Work out the finished part from the listing and answer in its coordinate system (mm). Face numbers are marked on the shaded views. A direction names the side the tool comes from. Coordinates: 2 decimals unless noted, no trailing zeros. Order: outer loops, then holes, each group sorted by start corner. A loop starts at its lowest first (then second) coordinate and runs counter-clockwise, first axis right, second up. Notation, with made-up numbers: (-31, 87) -> (28, 87) arc R25 cw to (28, 105) -> close; hole circle Ø3 at (35.25, -39.5). An arc over 180 degrees is marked (long way). Use one line per item in the form item = value.
Autodesk Inventor part; units mm, degrees
ref_plane "YZ Plane" through (0, 0, 0) normal (1, 0, 0) x (0, 1, 0)
ref_plane "XZ Plane" through (0, 0, 0) normal (0, 1, 0) x (-1, 0, 0)
ref_plane "XY Plane" through (0, 0, 0) normal (0, 0, 1) x (1, 0, 0)
sketch "Sketch1" plane through (0, 0, 0) normal (0, 1, 0) x (-1, 0, 0)
  circle A0 centre (0, 0) radius 47.5
  dimension "d0" = 95
extrude "Extrusion1" add sketch "Sketch1" along normal blind 6
sketch "Sketch2" plane through (0, 6, 0) normal (0, 1, 0) x (1, 0, 0)
  circle A0 centre (0, 0) radius 10
  circle A1 centre (0, 5) radius 1
  circle A2 centre (0, -5) radius 1
  dimension "d3" = 20
  dimension "d4" = 2
  dimension "d5" = 2
extrude "Extrusion2" cut sketch "Sketch2" against normal blind 23.4625 contours A1 | A2
sketch "Sketch4" plane through (0, 6, 0) normal (0, 1, 0) x (1, 0, 0)
  line L0 (0, 0) -> (-10, 0)
  line L1 (-10, 0) -> (-10, 25)
  line L2 (-10, 25) -> (0, 25)
  line L3 (0, 25) -> (0, 0)
  line L4 (0, 0) -> (-5, 0)
  line L5 (-5, 0) -> (-5, 25)
  line L6 (-5, 25) -> (0, 25)
  line L7 (0, 25) -> (0, 0)
  line L8 (-5, 25) -> (-20, 25)
  line L9 (-20, 25) -> (-20, -25)
  line L10 (-20, -25) -> (-5, -25)
  line L11 (-5, -25) -> (-5, 25)
  line L12 (-5, 25) -> (-25, 25)
  line L13 (-25, 25) -> (-25, -25)
  line L14 (-25, -25) -> (-5, -25)
  line L15 (-5, -25) -> (-5, 25)
  dimension "d9" = 10
  dimension "d10" = 25
  dimension "d11" = 15
  dimension "d12" = 50
  dimension "d13" = 20
extrude "Extrusion3" add sketch "Sketch4" along normal blind 70 contours L11 L10 L9 L8 L1 L0 | L0 L1 L2 L5 | L14 L13 L12 L9
sketch "Sketch5" plane through (-25, 6, -25) normal (-1, 0, 0) x (0, 0, 1)
  line L0 (0, 0) -> (0, 70)
  line L1 (50, 0) -> (50, 70)
  line L2 (0, 70) -> (50, 70)
  line L3 (50, 70) -> (50, 0)
  line L4 (50, 0) -> (0, 0)
  line L5 (0, 0) -> (0, 70)
  line L6 (50, 70) -> (0, 70)
  line L7 (72.5, 0) -> (-22.5, 0)
  line L8 (0, 70) -> (25, 70)
  line L9 (25, 70) -> (25, 0)
  line L10 (25, 0) -> (0, 0)
  line L11 (0, 0) -> (0, 70)
  line L12 (25, 35) -> (15, 35)
  line L13 (15, 35) -> (15, 15)
  line L14 (15, 15) -> (25, 15)
  line L15 (25, 15) -> (25, 35)
  line L16 (15, 35) -> (25, 35)
  line L17 (25, 35) -> (25, 55)
  line L18 (25, 55) -> (15, 55)
  line L19 (15, 55) -> (15, 35)
  line L20 (15, 15) -> (35, 15)
  line L21 (35, 15) -> (35, 55)
  line L22 (35, 55) -> (15, 55)
  line L23 (15, 55) -> (15, 15)
  line L24 (15, 15) -> (35, 15)
  line L25 (35, 15) -> (35, 55.5)
  line L26 (35, 55.5) -> (15, 55.5)
  line L27 (15, 55.5) -> (15, 15)
  point P0 (25, -6)
  dimension "d16" = 10
  dimension "d17" = 20
  dimension "d18" = 20
  dimension "d19" = 20
  dimension "d20" = 40.5
extrude "Extrusion4" cut sketch "Sketch5" against normal blind 16 contours L14 L13 L12 L9 | L9 L22 L21 L20 | L26 L25 L22 L9 | L9 L18 L27 L26 | L12 L19 L18 L9
sketch "Sketch6" plane through (-25, 6, -25) normal (-1, 0, 0) x (0, 0, 1)
  line L0 (35, 15) -> (15, 15)
  line L1 (15, 15) -> (35, 15)
  line L2 (35, 15) -> (35, 9)
  line L3 (35, 9) -> (15, 9)
  line L4 (15, 9) -> (15, 15)
  line L5 (15, 55.5) -> (35, 55.5)
  line L6 (15, 55.5) -> (35, 55.5)
  line L7 (35, 55.5) -> (35, 61.5)
  line L8 (35, 61.5) -> (15, 61.5)
  line L9 (15, 61.5) -> (15, 55.5)
  point P0 (25, -6)
  dimension "d23" = 6
  dimension "d24" = 6
extrude "Extrusion5" cut sketch "Sketch6" against normal blind 6
sketch "Sketch7" plane through (-19, 6, -25) normal (-1, 0, 0) x (0, 0, 1)
  line L0 (35, 9) -> (15, 9)
  line L1 (35, 61.5) -> (35, 9)
  line L2 (15, 9) -> (35, 9)
  line L3 (35, 9) -> (35, 11.6)
  line L4 (35, 11.6) -> (15, 11.6)
  line L5 (15, 11.6) -> (15, 9)
  line L6 (15, 55.5) -> (15, 61.5)
  line L7 (35, 61.5) -> (35, 55.5)
  line L8 (15, 61.5) -> (35, 61.5)
  line L9 (35, 61.5) -> (35, 58.5)
  line L10 (35, 58.5) -> (15, 58.5)
  line L11 (15, 58.5) -> (15, 61.5)
  line L12 (15, 9) -> (15, 61.5)
  line L13 (15, 9) -> (35, 9)
  line L14 (35, 9) -> (35, 12)
  line L15 (35, 12) -> (15, 12)
  line L16 (15, 12) -> (15, 9)
  line L17 (35, 15) -> (15, 15)
  line L18 (25, 15) -> (20, 15)
  line L19 (20, 15) -> (20, 12)
  line L20 (20, 12) -> (25, 12)
  line L21 (25, 12) -> (25, 15)
  line L22 (25, 15) -> (30, 15)
  line L23 (30, 15) -> (30, 12)
  line L24 (30, 12) -> (25, 12)
  line L25 (25, 12) -> (25, 15)
  line L26 (15, 61.5) -> (35, 61.5)
  line L27 (25, 58.5) -> (20, 58.5)
  line L28 (20, 58.5) -> (20, 61.5)
  line L29 (20, 61.5) -> (25, 61.5)
  line L30 (25, 61.5) -> (25, 58.5)
  line L31 (25, 58.5) -> (30, 58.5)
  line L32 (30, 58.5) -> (30, 61.5)
  line L33 (30, 61.5) -> (25, 61.5)
  line L34 (25, 61.5) -> (25, 58.5)
  circle A0 centre (20, 12) radius 1.35
  circle A1 centre (30, 12) radius 1.35
  circle A2 centre (20, 58.5) radius 1.35
  circle A3 centre (30, 58.5) radius 1.35
  point P0 (25, -6)
  dimension "d27" = 2.6
  dimension "d28" = 3
  dimension "d29" = 3
  dimension "d30" = 5
  dimension "d31" = 5
  dimension "d32" = 2.7
  dimension "d33" = 2.7
  dimension "d34" = 2.7
  dimension "d35" = 2.7
extrude "Extrusion6" cut sketch "Sketch7" against normal blind 10 contours A1 L4 | L4 A1 L15 | A0 L15 L4 | L4 A0 | L15 L23 A1 | A0 L19 L15 | L15 A1 L23 | L15 L19 A0 | A3 L10 | L10 L32 A3 | A2 L28 L10 | L10 A2 | L10 A3 L32 | L28 A2 L10
thread "Thread1"
thread "Thread2"
thread "Thread3"
thread "Thread4"
sketch "Sketch8" plane through (-9, 6, -25) normal (-1, 0, 0) x (0, 0, 1)
  line L0 (15, 9) -> (15, 61.5)
  line L1 (35, 55.5) -> (35, 15)
  line L2 (15, 61.5) -> (35, 61.5)
  line L3 (35, 61.5) -> (35, 44.5)
  line L4 (35, 44.5) -> (15, 44.5)
  line L5 (15, 44.5) -> (15, 61.5)
  circle A0 centre (25, 44.5) radius 10
  point P0 (25, -6)
  dimension "d46" = 17
  dimension "d47" = 20
extrude "Extrusion7" cut sketch "Sketch8" against normal blind 15.4 contours A0 L4 | L4 A0
sketch "Sketch9" plane through (0, 6, 0) normal (0, 1, 0) x (1, 0, 0)
  circle A0 centre (0, 0) radius 1.5
  dimension "d50" = 3
extrude "Extrusion8" cut sketch "Sketch9" against normal blind 15.4
sketch "Sketch10" plane through (0, 0, 0) normal (0, -1, 0) x (1, 0, 0)
  circle A0 centre (0, 0) radius 2.6
  dimension "d53" = 5.2
extrude "Extrusion9" cut sketch "Sketch10" against normal blind 3.65
sketch "Sketch11" plane through (-19, 6, -25) normal (-1, 0, 0) x (0, 0, 1)
  line L0 (15, 55.5) -> (15, 61.5)
  line L1 (35, 55.5) -> (35, 44.5)
  line L2 (15, 61.5) -> (35, 61.5)
  line L3 (35, 61.5) -> (35, 55.5)
  line L4 (35, 55.5) -> (15, 55.5)
  line L5 (15, 55.5) -> (15, 61.5)
  point P0 (25, -6)
extrude "Extrusion10" cut sketch "Sketch11" against normal blind 10
sketch "Sketch12" plane through (-9, 6, -25) normal (-1, 0, 0) x (0, 0, 1)
  line L0 (15, 61.5) -> (35, 61.5)
  line L1 (35, 61.5) -> (35, 9)
  line L2 (15, 61.5) -> (35, 61.5)
  line L3 (35, 61.5) -> (35, 58.5)
  line L4 (35, 58.5) -> (15, 58.5)
  line L5 (15, 58.5) -> (15, 61.5)
  line L6 (15, 61.5) -> (21, 61.5)
  line L7 (21, 61.5) -> (21, 58.5)
  line L8 (21, 58.5) -> (15, 58.5)
  line L9 (15, 58.5) -> (15, 61.5)
  line L10 (15, 61.5) -> (35, 61.5)
  line L11 (35, 61.5) -> (29, 61.5)
  line L12 (29, 61.5) -> (29, 58.5)
  line L13 (29, 58.5) -> (35, 58.5)
  line L14 (35, 58.5) -> (35, 61.5)
  point P0 (25, -6)
  dimension "d58" = 3
  dimension "d59" = 6
  dimension "d60" = 6
extrude "Extrusion11" add sketch "Sketch12" along normal blind 12 contours L0 L7 L4 L5 | L0 L1 L4 L12
sketch "Sketch13" plane through (-25, 6, -25) normal (-1, 0, 0) x (0, 0, 1)
  line L0 (15, 61.5) -> (35, 61.5)
  line L1 (35, 61.5) -> (35, 64.5)
  line L2 (35, 64.5) -> (15, 64.5)
  line L3 (15, 64.5) -> (15, 61.5)
  line L4 (15, 64.5) -> (12, 64.5)
  line L5 (12, 64.5) -> (12, 44.5)
  line L6 (12, 44.5) -> (15, 44.5)
  line L7 (15, 44.5) -> (15, 64.5)
  line L8 (35, 64.5) -> (38, 64.5)
  line L9 (38, 64.5) -> (38, 44.5)
  line L10 (38, 44.5) -> (35, 44.5)
  line L11 (35, 44.5) -> (35, 64.5)
  point P0 (25, -6)
  dimension "d63" = 20
  dimension "d64" = 3
  dimension "d65" = 3
  dimension "d66" = 20
  dimension "d67" = 3
extrude "Extrusion12" add sketch "Sketch13" along normal blind 30
sketch "Sketch16" plane through (-55, 6, -25) normal (-1, 0, 0) x (0, 0, 1)
  line L0 (12, 44.5) -> (15, 44.5)
  line L1 (38, 64.5) -> (12, 64.5)
  line L2 (12, 44.5) -> (15, 44.5)
  line L3 (15, 44.5) -> (15, 64.5)
  line L4 (15, 64.5) -> (12, 64.5)
  line L5 (12, 64.5) -> (12, 44.5)
  line L6 (38, 44.5) -> (38, 64.5)
  line L7 (12, 64.5) -> (38, 64.5)
  line L8 (38, 64.5) -> (38, 61.5)
  line L9 (38, 61.5) -> (12, 61.5)
  line L10 (12, 61.5) -> (12, 64.5)
  line L11 (35, 44.5) -> (38, 44.5)
  line L12 (38, 64.5) -> (35, 64.5)
  line L13 (35, 64.5) -> (35, 44.5)
  line L14 (35, 44.5) -> (38, 44.5)
  line L15 (38, 44.5) -> (38, 64.5)
  point P0 (25, -6)
  point P1 (15, 61.5)
  point P2 (35, 61.5)
  dimension "d70" = 3
  dimension "d71" = 3
extrude "Extrusion13" add sketch "Sketch16" along normal blind 3
sketch "Sketch17" plane through (-19, 21, -10) normal (0, 0, 1) x (1, 0, 0)
  line L0 (-39, 46.5) -> (-2, 46.5)
  line L1 (-6, 29.5) -> (-39, 29.5)
  line L2 (-39, 46.5) -> (-36, 46.5)
  line L3 (-36, 46.5) -> (-36, 29.5)
  line L4 (-36, 29.5) -> (-39, 29.5)
  line L5 (-39, 29.5) -> (-39, 46.5)
  point P0 (19, -21)
  dimension "d74" = 3
extrude "Extrusion14" add sketch "Sketch17" along normal blind 20
sketch "Sketch19" plane through (-25, 70.5, 13) normal (0, 1, 0) x (1, 0, 0)
  line L0 (0, 26) -> (-33, 26)
  line L1 (0, 26) -> (-10.9488, 26)
  line L2 (-10.9488, 26) -> (-10.9488, 13)
  line L3 (-10.9488, 13) -> (0, 13)
  line L4 (0, 13) -> (0, 26)
  line L5 (0, 13) -> (-12, 13)
  line L6 (-12, 13) -> (-12, 17)
  line L7 (-12, 17) -> (0, 17)
  line L8 (0, 17) -> (0, 13)
  line L9 (0, 26) -> (0, 0)
  line L10 (-12, 13) -> (0, 13)
  line L11 (0, 13) -> (0, 9)
  line L12 (0, 9) -> (-12, 9)
  line L13 (-12, 9) -> (-12, 13)
  point P0 (25, 13)
  dimension "d77" = 12
  dimension "d78" = 4
  dimension "d79" = 4
extrude "Extrusion15" cut sketch "Sketch19" against normal blind 4 contours L4 L3 L2 L7 | L2 L5 L6 L7 | L9 L12 L13 L5 L3
sketch "Sketch20" plane through (-21, 6, -25) normal (-1, 0, 0) x (0, 0, 1)
  line L0 (15, 58.5) -> (21, 58.5)
  line L1 (15, 61.5) -> (21, 61.5)
  line L2 (15, 58.5) -> (21, 58.5)
  line L3 (21, 58.5) -> (21, 61.5)
  line L4 (21, 61.5) -> (15, 61.5)
  line L5 (15, 61.5) -> (15, 58.5)
  line L6 (29, 61.5) -> (35, 61.5)
  line L7 (29, 61.5) -> (35, 61.5)
  line L8 (35, 61.5) -> (35, 58.5)
  line L9 (35, 58.5) -> (29, 58.5)
  line L10 (29, 58.5) -> (29, 61.5)
  point P0 (25, -6)
extrude "Extrusion16" cut sketch "Sketch20" against normal blind 3
properties part number "Base top w servo housing"
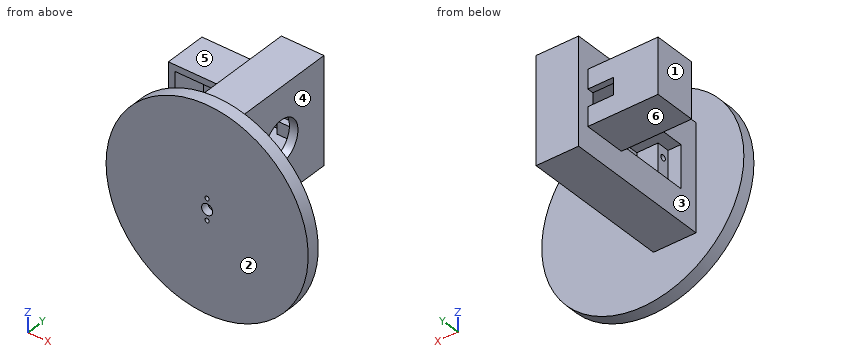
(1) Each of these flat-tipped pins is pushed along its axis until it touches: P1, Ø6, axis at x = -26.5, y = 9.5, coming from the -Z side; P2, Ø2.5, axis at y = 18, z = -5, coming from the -X side; P3, Ø7, axis at x = 0, z = 0, coming from the +Y side. Where does it stop, or does it pass through?
Data:
P1 = -25
P2 = -9
P3 = 6
(2) Section B-B on x = -40.5 is taken. Write down the section's boundary in (y, z).
Data:
outline = (0, -24.82) -> (6, -24.82) -> (6, 24.82) -> (0, 24.82) -> close; (50.5, -13) -> (70.5, -13) -> (70.5, 13) -> (50.5, 13) -> (50.5, 10) -> (67.5, 10) -> (67.5, -10) -> (50.5, -10) -> close
(3) Section A-A on z = 0 is taken. Count the separate pieces of the cut face and the enclosed holes in it, plus the area to 3 significant figures.
Data:
separate_pieces = 4
enclosed_holes = 0
area = 1,200 mm²
(4) The mould has two halves that part along Y. Classify the marked faces 1, 2 and 3: released by +Y, released by -Y, zero draft, split by the parting line, or undercut.
Data:
face_1 = zero draft
face_2 = released by -Y
face_3 = undercut
(5) Which of the six approach directions +Z, -Z, +X, -X, +Y, -Y give full straight-line access (tool end or side, diameter ignored) to the marked faces 4, 5 and 6?
Data:
face_4 = +Z, -Z, +X, +Y
face_5 = +Z, -X, +Y
face_6 = -Z, -X, +Y
(6) Straight lines are drawn through the part: line 1 along Y through (x, z) = (-14, 5); line 2 along Z through (x, y) = (-14, 18); line 3 along Y through (x, z) = (-29.5, 12.5). For each, find the intervals that lie inside material, in ascending order.
Data:
line_1 = 0 to 16.65, 19.35 to 21, 64.5 to 76
line_2 = -25 to -6.35, -3.65 to 3.65, 6.35 to 25
line_3 = 0 to 6, 50.5 to 70.5
(7) Section D-D on x = -21 is taken. Write down the section's boundary in (y, z).
Data:
outline = (0, -42.61) -> (6, -42.61) -> (6, -25) -> (76, -25) -> (76, 25) -> (6, 25) -> (6, 42.61) -> (0, 42.61) -> close; hole (15, -10) -> (67.5, -10) -> (67.5, 10) -> (15, 10) -> close
(8) Section C-C on y = 38 is taken. Write down the section's boundary in (x, z), plus the area to 3 significant figures.
Data:
outline = (-25, -25) -> (-5, -25) -> (-5, 25) -> (-25, 25) -> (-25, 10) -> (-9, 10) -> (-9, -10) -> (-25, -10) -> close
area = 680 mm²
